```python
from build123d import *

# Parameters (mm, degrees)
SKETCH1_R           = 11
BOSS_EXTRUDE1_DEPTH = 10
SKETCH2_R           = 11
SKETCH2_R_2         = 4.125
BOSS_EXTRUDE2_DEPTH = 2.5
SKETCH4_R           = 2
SKETCH4_R_2         = 11.5
CUT_EXTRUDE1_DEPTH  = 10
BOSS_EXTRUDE3_DEPTH = 10
BOSS_EXTRUDE4_DEPTH = 10
FILLET1_R           = 25
CUT_EXTRUDE5_DEPTH  = 10
BOSS_EXTRUDE6_DEPTH = 10
FILLET3_R           = 25
BOSS_EXTRUDE7_DEPTH = 10
FILLET4_R           = 25


with BuildPart() as part:
    # Sketch1 → Boss-Extrude1 (new body)
    with BuildSketch(Plane(origin=(0, 0, 0), x_dir=(1, 0, 0), z_dir=(0, 1, 0))):
        with BuildLine():
            Line((-45, -27), (-25, -27))
            Line((-25, -27), (25, -27))
            Line((25, -27), (45, -27))
            Line((45, -27), (70, -27))
            Line((70, -27), (70, -2))
            Line((70, -2), (70, 0))
            ThreePointArc((70, 0), (62.67766953, 17.67766953), (45, 25))
            Line((45, 25), (-45, 25))
            ThreePointArc((-45, 25), (-62.67766953, 17.67766953), (-70, 0))
            Line((-70, 0), (-70, -2))
            Line((-70, -2), (-70, -27))
            Line((-70, -27), (-45, -27))
        make_face()
        with Locations(Location((-45, 0, 0), (0, 0, 90))):  # turned: the seam where the file's is
            Circle(SKETCH1_R, mode=Mode.SUBTRACT)
        with Locations(Location((45, 0, 0), (0, 0, 270))):  # turned: the seam where the file's is
            Circle(SKETCH1_R, mode=Mode.SUBTRACT)
    extrude(amount=BOSS_EXTRUDE1_DEPTH)

    # Sketch2 → Boss-Extrude2 (add)
    with BuildSketch(Plane.XZ):
        with Locations(Location((45, 0, 0), (0, 0, 270))):  # turned: the seam where the file's is
            Circle(SKETCH2_R)
        with Locations(Location((45, 0, 0), (0, 0, 270))):  # turned: the seam where the file's is
            Circle(SKETCH2_R_2, mode=Mode.SUBTRACT)
        with Locations(Location((-45, 0, 0), (0, 0, 270))):  # turned: the seam where the file's is
            Circle(SKETCH2_R)
        with Locations(Location((-45, 0, 0), (0, 0, 270))):  # turned: the seam where the file's is
            Circle(SKETCH2_R_2, mode=Mode.SUBTRACT)
    extrude(amount=-BOSS_EXTRUDE2_DEPTH)

    # Sketch4 → Cut-Extrude1 (cut)
    with BuildSketch(Plane(origin=(0, 10, 0), x_dir=(1, 0, 0), z_dir=(0, 1, 0))):
        with Locations(Location((15.5, 15.5, 0), (0, 0, 270))):  # turned: the seam where the file's is
            Circle(SKETCH4_R)
        with Locations(Location((-15.5, 15.5, 0), (0, 0, 270))):  # turned: the seam where the file's is
            Circle(SKETCH4_R)
        with Locations(Location((-15.5, -15.5, 0), (0, 0, 270))):  # turned: the seam where the file's is
            Circle(SKETCH4_R)
        with Locations(Location((15.5, -15.5, 0), (0, 0, 270))):  # turned: the seam where the file's is
            Circle(SKETCH4_R)
        with Locations(Location((0, 0, 0), (0, 0, 270))):  # turned: the seam where the file's is
            Circle(SKETCH4_R_2)
    extrude(amount=-CUT_EXTRUDE1_DEPTH, mode=Mode.SUBTRACT)

    # Sketch5 → Boss-Extrude3 (add)
    with BuildSketch(Plane(origin=(0, 0, 0), x_dir=(-1, 0, 0), z_dir=(0, -1, 0))):
        Polygon((-70, -27), (-151.373495533, -27), (-151.373495533, 25), (-45, 25), (-50.986838326, 16.31487445), (-65.445821875, 2.682118533), (-66.139224666, -20.893576385), align=None)
    extrude(amount=-BOSS_EXTRUDE3_DEPTH)

    # Sketch6 → Boss-Extrude4 (add)
    with BuildSketch(Plane(origin=(0, 0, 0), x_dir=(-1, 0, 0), z_dir=(0, -1, 0))):
        Polygon((-151.373495533, 25), (-170, 25), (-170, -27), (-151.373495533, -27), (-141.038307318, -1), align=None)
    extrude(amount=-BOSS_EXTRUDE4_DEPTH)

    # Fillet1
    fillet1_edges = [part.edges().sort_by_distance(p)[0] for p in [
        (170, 5, 27),
        (170, 5, -25),
        (-70, 5, 27),
    ]]
    fillet(fillet1_edges, radius=FILLET1_R)

    # Sketch7 → Cut-Extrude5 (cut)
    with BuildSketch(Plane(origin=(0, 10, 0), x_dir=(1, 0, 0), z_dir=(0, 1, 0))):
        with BuildLine():
            Line((133.980635502, -69.297657421), (165.367779164, -26))
            Line((165.367779164, -26), (152, -26))
            ThreePointArc((152, -26), (148.535533906, -26.748737342), (145, -27))
            Line((145, -27), (-45, -27))
            ThreePointArc((-45, -27), (-48.535533906, -26.748737342), (-52, -26))
            Line((-52, -26), (-59.265699986, -26))
            Line((-59.265699986, -26), (-45.110713629, -66.528203569))
            Line((-45.110713629, -66.528203569), (133.980635502, -69.297657421))
        make_face()
        with BuildLine():
            ThreePointArc((145, -27), (148.535533906, -26.748737342), (152, -26))
            Line((152, -26), (-52, -26))
            ThreePointArc((-52, -26), (-48.535533906, -26.748737342), (-45, -27))
            Line((-45, -27), (145, -27))
        make_face()
    extrude(amount=-CUT_EXTRUDE5_DEPTH, mode=Mode.SUBTRACT)

    # Sketch10 → Boss-Extrude6 (add)
    with BuildSketch(Plane(origin=(0, 10, 0), x_dir=(1, 0, 0), z_dir=(0, 1, 0))):
        with BuildLine():
            Line((-63.907316272, 7.976406282), (-70, 0))
            ThreePointArc((-70, 0), (-62.67766953, 17.67766953), (-45, 25))
            Line((-45, 25), (145, 25))
            ThreePointArc((145, 25), (162.67766953, 17.67766953), (170, 0))
            Line((170, 0), (55.598298081, 15.952812565))
            Line((55.598298081, 15.952812565), (0, 23.705749919))
            Line((0, 23.705749919), (-30.230523, 19.829281242))
            Line((-30.230523, 19.829281242), (-63.907316272, 7.976406282))
        make_face()
        with BuildLine():
            Line((-70, 0), (-70, 26))
            Line((-70, 26), (170, 26))
            Line((170, 26), (170, 0))
            ThreePointArc((170, 0), (162.67766953, 17.67766953), (145, 25))
            Line((145, 25), (-45, 25))
            ThreePointArc((-45, 25), (-62.67766953, 17.67766953), (-70, 0))
        make_face()
    extrude(amount=-BOSS_EXTRUDE6_DEPTH)

    # Fillet3
    fillet3_edges = [part.edges().sort_by_distance(p)[0] for p in [
        (-70, 5, -26),
        (170, 5, -26),
    ]]
    fillet(fillet3_edges, radius=FILLET3_R)

    # Sketch11 → Boss-Extrude7 (add)
    with BuildSketch(Plane(origin=(0, 10, 0), x_dir=(1, 0, 0), z_dir=(0, 1, 0))):
        with BuildLine():
            Line((170, -2), (170, -0.5))
            Line((170, -0.5), (142.437846572, -19.831941741))
            Line((142.437846572, -19.831941741), (-54.330276999, -19.831941741))
            Line((-54.330276999, -19.831941741), (-70, -0.5))
            Line((-70, -0.5), (-70, -2))
            ThreePointArc((-70, -2), (-65, -17), (-52, -26))
            Line((-52, -26), (152, -26))
            ThreePointArc((152, -26), (165, -17), (170, -2))
        make_face()
        with BuildLine():
            Line((170, -26.5), (170, -2))
            ThreePointArc((170, -2), (165, -17), (152, -26))
            Line((152, -26), (-52, -26))
            ThreePointArc((-52, -26), (-65, -17), (-70, -2))
            Line((-70, -2), (-70, -26.5))
            Line((-70, -26.5), (170, -26.5))
        make_face()
    extrude(amount=-BOSS_EXTRUDE7_DEPTH)

    # Fillet4
    fillet4_edges = [part.edges().sort_by_distance(p)[0] for p in [
        (-70, 5, 26.5),
        (170, 5, 26.5),
    ]]
    fillet(fillet4_edges, radius=FILLET4_R)


solid = part.part
```
For this review, take the finished solid that the model builds, in its own axes (mm). A direction names the side the tool comes from. Round coordinates to 2 decimals unless told otherwise and drop trailing zeros. Loops run counter-clockwise (first coordinate to the right, second up) from the corner with the lowest first, then second, coordinate; pieces in that order, holes last.
Q1. Mouldability with a two-part tool opening along Z and no side actions: class faces 1 (the face through (-49, 1, 1)), 2 (the face through (162.482, 4.93, -18.871)), 3 (the face through (52, 10, 12)) as +Z half, -Z half, draft (parallel to the pull), parting line (faces both ways), or undercut.
Result sheet:
face 1: undercut
face 2: -Z half
face 3: draft
Q2. Add section D-D on z = -15.5. Write out the cut boundary in (x, y).
Result sheet:
outline: (-65.37, 0) - (-17.5, 0) - (-17.5, 10) - (-65.37, 10) - close; (-13.5, 0) - (13.5, 0) - (13.5, 10) - (-13.5, 10) - close; (17.5, 0) - (165.37, 0) - (165.37, 10) - (17.5, 10) - close
Q3. Add section A-A on x = -15.5. Write out the cut boundary in (y, z).
Result sheet:
outline: (0, -26) - (10, -26) - (10, -17.5) - (0, -17.5) - close; (0, -13.5) - (10, -13.5) - (10, 13.5) - (0, 13.5) - close; (0, 17.5) - (10, 17.5) - (10, 26.5) - (0, 26.5) - close
Q4. Insertion check: pin 1 Ø5 at (y, z) = (5, -11) entering from +X; pin 2 Ø2 at (y, z) = (6, 3) entering from +X (3 decimals); pin 3 Ø3 at (y, z) = (5.5, -19.5) entering from -X; pin 4 Ø24 at (x, z) = (-46, -4.5) entering from +Y. Each pin has a flat end and moves straight along its axis. Give the tip position at first contact, or say it passes through.
Result sheet:
pin 1: stops at x = 168.85
pin 2: stops at x = 169.995
pin 3: stops at x = -63.33
pin 4: stops at y = 10
Q5. Machinability: for faces 4 (the face through (17.483, 5.07, 15.24)), 5 (the face through (55.906, 6.198, -1.432)), which of the approach directions +Z, -Z, +X, -X, +Y, -Y give a long, thin tool a straight path to every point of the face, cutting with its end or side? Answer none if there is none.
Result sheet:
face 4: +Y, -Y
face 5: +Y
Q6. Add section C-C on x = 45. Write out the cut boundary in (y, z) (3 decimals), plus the area to 3 significant figures.
Result sheet:
outline: (0, -26) - (10, -26) - (10, -11) - (2.5, -11) - (2.5, -4.125) - (0, -4.125) - close; (0, 4.125) - (2.5, 4.125) - (2.5, 11) - (10, 11) - (10, 26.5) - (0, 26.5) - close
area: 339 mm2
Q7. Add section B-B on y = 4.5. Write out the cut boundary in (x, z), plus the area to 3 significant figures.
Result sheet:
outline: (-70, -1) arc R25 ccw to (-45, -26) - (145, -26) arc R25 ccw to (170, -1) - (170, 1.5) arc R25 ccw to (145, 26.5) - (-45, 26.5) arc R25 ccw to (-70, 1.5) - close; hole circle Ø22 at (-45, 0); hole circle Ø4 at (-15.5, -15.5); hole circle Ø4 at (-15.5, 15.5); hole circle Ø23 at (0, 0); hole circle Ø4 at (15.5, -15.5); hole circle Ø4 at (15.5, 15.5); hole circle Ø22 at (45, 0)
area: 10,800 mm2
Q8. To check wall thickness, follow line 1 along X through (y, z) = (6.5, 0); line 2 along X through (y, z) = (1.7, 0) (3 decimals); line 3 along Y through (x, z) = (-51, -9). State the ranges of each line that lie inside material, in increasing order.
Result sheet:
line 1: x = -70 to -56, -34 to -11.5, 11.5 to 34, 56 to 170
line 2: x = -70 to -49.125, -40.875 to -11.5, 11.5 to 40.875, 49.125 to 170
line 3: y = 0 to 2.5
